CAD build for the part. Positions are in the model's coordinates, mm. A direction names the side the tool comes from. Coordinates: 2 decimals unless noted, no trailing zeros. Order: outer loops, then holes, each group sorted by start corner. A loop starts at its lowest first (then second) coordinate and runs counter-clockwise, first axis right, second up. Notation, with made-up numbers: M 38,6 L 51,6 A23 cw 51,21 Z; hole C 70.25,69.25 d7. An arc over 180 degrees is marked long. One line per item, written item: value.
from build123d import *

# Parameters (mm, degrees)
BOSS_EXTRUDE1_DEPTH = 2.54
SKETCH1_7_W         = 5.08
SKETCH1_7_H         = 2.032
BOSS_EXTRUDE2_DEPTH = 17.272
SKETCH2_W           = 5.08
SKETCH2_H           = 17.272
BOSS_EXTRUDE3_DEPTH = 2.54
SKETCH3_R           = 1.27
BOSS_EXTRUDE4_DEPTH = 8.89
FILLET1_R           = 0.635
SKETCH4_R           = 1.27
BOSS_EXTRUDE5_DEPTH = 1.27


with BuildPart() as part:
    # Sketch1 → Boss-Extrude1 (new body)
    with BuildSketch(Plane.XY):
        with BuildLine():
            ThreePointArc((-78.760738581, 73.886338755), (-81.300738581, 71.346338755), (-83.840738581, 73.886338755))
            Line((-83.840738581, 73.886338755), (-83.840738581, 69.568338755))
            Line((-83.840738581, 69.568338755), (-78.760738581, 69.568338755))
            Line((-78.760738581, 69.568338755), (-78.760738581, 73.886338755))
        make_face()
        with BuildLine():
            ThreePointArc((-78.760738581, 73.886338755), (-81.300738581, 76.426338755), (-83.840738581, 73.886338755))
            Line((-83.840738581, 73.886338755), (-78.760738581, 73.886338755))
        make_face()
        with BuildLine():
            Line((-78.760738581, 73.886338755), (-83.840738581, 73.886338755))
            ThreePointArc((-83.840738581, 73.886338755), (-81.300738581, 71.346338755), (-78.760738581, 73.886338755))
        make_face()
        with BuildLine():
            ThreePointArc((-78.760738581, 47.978338755), (-81.300738581, 50.518338755), (-83.840738581, 47.978338755))
            Line((-83.840738581, 47.978338755), (-78.760738581, 47.978338755))
        make_face()
        with BuildLine():
            Line((-78.760738581, 47.978338755), (-83.840738581, 47.978338755))
            ThreePointArc((-83.840738581, 47.978338755), (-81.300738581, 45.438338755), (-78.760738581, 47.978338755))
        make_face()
        with BuildLine():
            Line((-78.760738581, 52.296338755), (-83.840738581, 52.296338755))
            Line((-83.840738581, 52.296338755), (-83.840738581, 47.978338755))
            ThreePointArc((-83.840738581, 47.978338755), (-81.300738581, 50.518338755), (-78.760738581, 47.978338755))
            Line((-78.760738581, 47.978338755), (-78.760738581, 52.296338755))
        make_face()
    extrude(amount=BOSS_EXTRUDE1_DEPTH)

    # Sketch1<7> → Boss-Extrude2 (add)
    with BuildSketch(Plane.XY):
        with Locations((-81.300738581, 53.312338755)):
            Rectangle(SKETCH1_7_W, SKETCH1_7_H)
        Polygon((-78.760738581, 69.568338755), (-83.840738581, 69.568338755), (-83.840738581, 67.536338755), (-82.574456105, 67.536338755), (-78.760738581, 67.536338755), align=None)
    extrude(amount=BOSS_EXTRUDE2_DEPTH)

    # Sketch2 → Boss-Extrude3 (add)
    with BuildSketch(Plane.XY.offset(17.272)):
        with Locations((-81.300738581, 60.932338755)):
            Rectangle(SKETCH2_W, SKETCH2_H)
    extrude(amount=BOSS_EXTRUDE3_DEPTH)

    # Sketch3 → Boss-Extrude4 (add)
    with BuildSketch(Plane.XY.offset(19.812)):
        with Locations(Location((-81.300738581, 60.932338755, 0), (0, 0, 180))):
            Circle(SKETCH3_R)
    extrude(amount=BOSS_EXTRUDE4_DEPTH)

    # Fillet1
    fillet1_edges = [part.edges().sort_by_distance(p)[0] for p in [
        (-81.300738581, 76.426338755, 2.54),
        (-83.840738581, 71.727338755, 2.54),
        (-78.760738581, 69.568338755, 11.176),
        (-83.840738581, 69.568338755, 11.176),
        (-81.300738581, 69.568338755, 2.54),
        (-83.840738581, 52.296338755, 11.176),
        (-78.760738581, 60.932338755, 19.812),
        (-78.760738581, 52.296338755, 11.176),
        (-81.300738581, 69.568338755, 19.812),
        (-81.300738581, 52.296338755, 19.812),
        (-83.840738581, 60.932338755, 19.812),
        (-81.300738581, 45.438338755, 2.54),
        (-83.840738581, 50.137338755, 2.54),
        (-78.760738581, 50.137338755, 2.54),
        (-81.300738581, 52.296338755, 2.54),
        (-78.760738581, 71.727338755, 2.54),
        (-80.030738581, 60.932338755, 19.812),
    ]]
    fillet(fillet1_edges, radius=FILLET1_R - 0.0001)  # a hair under: the kernel refuses the full size

    # Sketch4 → Boss-Extrude5 (add)
    with BuildSketch(Plane(origin=(0, 0, 0), x_dir=(-1, 0, 0), z_dir=(0, 0, -1))):
        with Locations(Location((81.300738581, 73.886338755, 0), (0, 0, 180))):
            Circle(SKETCH4_R)
        with Locations(Location((81.300738581, 47.978338755, 0), (0, 0, 180))):
            Circle(SKETCH4_R)
    extrude(amount=BOSS_EXTRUDE5_DEPTH)


solid = part.part
Q1. Slice it at B-B (y = 72). List the corners of the cut face in (x, z).
Recorded:
outline: M -83.84,0 L -78.76,0 L -78.76,1.91 A0.63 ccw -79.4,2.54 L -83.21,2.54 A0.63 ccw -83.84,1.91 Z
Q2. Mould opens along Y. For faces 6 (the face through (-81.36, 45.44, 0.94)), 7 (the face through (-81, 61, 17.272)), 8 (the face through (-81, 49, 2.54)) say: released by +Y, released by -Y, zero draft, split by the parting line, or undercut.
Recorded:
face 6: released by -Y
face 7: undercut
face 8: zero draft
Q3. Slice it at A-A (z = 7.25). List the corners of the cut face in (x, y).
Recorded:
outline: M -83.84,52.93 A0.63 ccw -83.21,52.3 L -79.4,52.3 A0.63 ccw -78.76,52.93 L -78.76,54.33 L -83.84,54.33 Z; M -83.84,67.54 L -78.76,67.54 L -78.76,68.93 A0.63 ccw -79.4,69.57 L -83.21,69.57 A0.63 ccw -83.84,68.93 Z
Q4. Slice it at C-C (z = 25.5). List the corners of the cut face in (x, y), plus the area to 3 significant figures.
Recorded:
outline: C -81.3,60.93 d2.54
area: 5.07 mm^2
Q5. Drill centre lines: line 1 along Y through (x, z) = (-79.8, 17); line 2 along Z through (x, y) = (-81.25, 61.5); line 3 along Z through (x, y) = (-82.4, 55). Where is each one in solid material? Low to high.
Recorded:
line 1: y = 52.3 to 54.33, 67.54 to 69.57
line 2: z = 17.27 to 28.7
line 3: z = 17.27 to 19.81
Q6. Pin check, flat tips, straight feed: pin 1 Ø2 at (x, z) = (-80, 17.5) entering from -Y; pin 2 Ø5 at (y, z) = (55, 11.5) entering from -X; pin 3 Ø3 at (x, z) = (-81.5, 7.5) entering from +Y; pin 4 Ø2.5 at (x, y) = (-82, 71) entering from -Z. Stop position of each tip, or through.
Recorded:
pin 1: stops at y = 52.3
pin 2: stops at x = -83.84
pin 3: stops at y = 69.57
pin 4: stops at z = 0
Q7. Which spindle directions (+Z, -Z, +X, -X, +Y, -Y) get a long thin tool onto all of the face, cutting with end or side? Do faces 1 (the face through (-81, 73, 2.54)), 2 (the face through (-82.24, 73.03, -0.63)), 3 (the face through (-81, 52.296, 11)), 4 (the face through (-81, 67.536, 9)), 5 (the face through (-80.03, 60.88, 24.52)). Say none if no direction does.
Recorded:
face 1: +Z, +X, -X, +Y
face 2: -Z
face 3: +Z, +X, -X, -Y
face 4: -Z, +X, -X
face 5: +Z
